Autodesk Inventor part; units mm, degrees
ref_plane "YZ Plane" through (0, 0, 0) normal (1, 0, 0) x (0, 1, 0)
ref_plane "XZ Plane" through (0, 0, 0) normal (0, 1, 0) x (-1, 0, 0)
ref_plane "XY Plane" through (0, 0, 0) normal (0, 0, 1) x (1, 0, 0)
sketch "Sketch1" plane through (0, 0, 0) normal (0, 0, 1) x (1, 0, 0)
  line L0 (0, 0) -> (203.2, 0)
  line L1 (152.5934, 101.6) -> (50.8, 101.6)
  line L2 (101.6, 0) -> (76.2, 0) construction
  line L3 (127, 101.6) -> (152.5934, 101.6)
  line L4 (0, 0) -> (3.175, 0) construction
  line L5 (152.5934, 101.6) -> (203.2, 0)
  line L6 (50.8, 101.6) -> (0, 0)
  line L7 (52.5749, 98.425) -> (52.6684, 98.2373)
  line L8 (31.4673, 0) -> (31.4673, 3.175) construction
  line L9 (31.4673, 3.175) -> (5.1373, 3.175)
  line L10 (22.7402, 38.3809) -> (5.1373, 3.175)
  line L11 (5.1373, 3.175) -> (51.6882, 96.6446)
  line L12 (176.1115, 47.2628) -> (198.0715, 3.175)
  line L13 (176.1115, 47.2628) -> (151.5146, 96.6447)
  line L14 (54.3484, 98.425) -> (148.8543, 98.425)
  line L15 (66.9801, 65.9439) -> (98.245, 3.175) construction
  line L16 (98.245, 3.175) -> (51.6882, 96.6446)
  line L17 (69.822, 67.3595) -> (54.3484, 98.425)
  line L18 (69.822, 67.3595) -> (101.6, 3.5605)
  line L19 (129.9466, 60.4672) -> (148.8543, 98.425)
  line L20 (132.7885, 59.0516) -> (151.5146, 96.6447)
  line L21 (148.8543, 98.425) -> (101.6, 3.5605)
  line L22 (132.7885, 59.0516) -> (104.9551, 3.175)
  line L23 (98.245, 3.175) -> (31.4673, 3.175)
  line L24 (201.6185, 3.175) -> (104.9551, 3.175)
  dimension "d0" = 203.2
  dimension "d40" = 3.175
  dimension "d42" = 3.175
  dimension "d44" = 3.175
  dimension "d45" = 3.175
  dimension "d51" = 101.6
  dimension "d52" = 93.4696
  dimension "d53" = 94.5059
  dimension "d54" = 96.6634
extrude "Extrusion2" add sketch "Sketch1" along normal blind 3.175
properties part number "Truss 3Tri"
Input: part model. Units: mm. Frame: model coordinates. A direction names the side the tool comes from. Give positions to 0.01 mm unless a question says otherwise; leave off trailing zeros. Loops run counter-clockwise (first coordinate to the right, second up) from the corner with the lowest first, then second, coordinate; pieces in that order, holes last. Notation, with made-up numbers: (64, 72) -> (97, 72) arc R18 cw to (97, 87) -> close; hole circle Ø10 at (-10.5, 50). An arc over 180 degrees is marked (long way). Use a Markdown table: item, result.
Q1. Section query C-C, the plane z = 1.05. Return the cut outline in (x, y) (1 decimal).
Entries:
| item | result |
|---|---|
| outline | (0, 0) -> (203.2, 0) -> (152.6, 101.6) -> (50.8, 101.6) -> close; hole (5.1, 3.2) -> (98.2, 3.2) -> (51.7, 96.6) -> close; hole (54.3, 98.4) -> (69.8, 67.4) -> (101.6, 3.6) -> (148.9, 98.4) -> close; hole (105, 3.2) -> (198.1, 3.2) -> (176.1, 47.3) -> (151.5, 96.6) -> (132.8, 59.1) -> close |
Q2. First-contact query: P1, Ø1, axis at x = 115.5, z = 1.5, coming from the -Y side; P2, Ø1.6, axis at x = 41.5, z = 2, coming from the +Y side. Flat tips, straight axial feed; report the tip coordinate or a pass-through.
Entries:
| item | result |
|---|---|
| P1 | stops at y = 0 |
| P2 | stops at y = 84.6 |
Q3. Section query D-D, the plane x = 91. Return the cut outline in (y, z) (3 decimals), plus the area to 3 significant figures.
Entries:
| item | result |
|---|---|
| outline | (0, 0) -> (3.175, 0) -> (3.175, 3.175) -> (0, 3.175) -> close; (17.72, 0) -> (24.842, 0) -> (24.842, 3.175) -> (17.72, 3.175) -> close; (98.425, 0) -> (101.6, 0) -> (101.6, 3.175) -> (98.425, 3.175) -> close |
| area | 42.8 mm² |
Q4. Access query for faces 1 (the flat face through (28.09, 49.26, 1.57)), 2 (the flat face through (116, 32, 0)). Directions: +Z, -Z, +X, -X, +Y, -Y. A direction counts if a zero-diameter tool reaches every point of the face in a straight line with its end or side. Return the directions, or none.
Entries:
| item | result |
|---|---|
| face 1 | +Z, -Z |
| face 2 | -Z, +X, -X, +Y, -Y |
Q5. Section query A-A, the plane y = 41. Return the cut outline in (x, z) (3 decimals).
Entries:
| item | result |
|---|---|
| outline | (20.5, 0) -> (23.975, 0) -> (23.975, 3.175) -> (20.5, 3.175) -> close; (79.405, 0) -> (82.952, 0) -> (82.952, 3.175) -> (79.405, 3.175) -> close; (120.25, 0) -> (123.797, 0) -> (123.797, 3.175) -> (120.25, 3.175) -> close; (179.231, 0) -> (182.778, 0) -> (182.778, 3.175) -> (179.231, 3.175) -> close |
Q6. Pull-direction query (X, two-part tool) for faces 3 (the flat face through (75.29, 49.26, 1.57)), 4 (the flat face through (116, 32, 3.175)), 5 (the flat face through (26, 52, 2)); classes: pulls with the +X half, pulls with the -X half, needs draft (parallel to the pull), parting line crosses it, or undercut.
Entries:
| item | result |
|---|---|
| face 3 | undercut |
| face 4 | needs draft |
| face 5 | pulls with the -X half |
Q7. Section query B-B, the plane x = 21.5. Return the cut outline in (y, z) (3 decimals).
Entries:
| item | result |
|---|---|
| outline | (0, 0) -> (3.175, 0) -> (3.175, 3.175) -> (0, 3.175) -> close; (36.03, 0) -> (43, 0) -> (43, 3.175) -> (36.03, 3.175) -> close |
Q8. Ray query, probe 1 along X at (y, z) = (49.5, 0.8); probe 2 along Y at (x, z) = (147, 1.35) (3 decimals); probe 3 along X at (y, z) = (17.5, 1.8). Return the intervals inside material, ascending. Write a range as from..to.
Entries:
| item | result |
|---|---|
| probe 1 | x = 24.75..28.21, 75.17..78.72, 124.48..128.03, 175..178.54 |
| probe 2 | y = 0..3.175, 87.582..94.702, 98.425..101.6 |
| probe 3 | x = 8.75..12.27, 91.11..94.66, 108.54..112.09, 190.94..194.48 |
